from build123d import *

# Parameters (mm, degrees)
SKETCH_1_W          = 20
SKETCH_1_H          = 19.5
EXTRUDE_1_DEPTH     = 4
SKETCH_2_W          = 20
SKETCH_2_H          = 5
EXTRUDE_2_DEPTH     = 21
SKETCH_3_W          = 9.5
SKETCH_3_H          = 7
EXTRUDE_3_DEPTH     = 3
SKETCH_4_W          = 9.5
SKETCH_4_H          = 7
EXTRUDE_4_DEPTH     = 3
SKETCH_5_R          = 2.6
CUT_EXTRUDE_1_DEPTH = 36.089172119
SKETCH_6_R          = 2.6
CUT_EXTRUDE_2_DEPTH = 30.791987178


with BuildPart() as part:
    # 草图1 → 凸台-拉伸1 (new body)
    with BuildSketch(Plane.XY):
        Rectangle(SKETCH_1_W, SKETCH_1_H)
    extrude(amount=EXTRUDE_1_DEPTH)

    # 草图2 → 凸台-拉伸2 (add)
    with BuildSketch(Plane.XY.offset(4)):
        with Locations((0, 7.25)):
            Rectangle(SKETCH_2_W, SKETCH_2_H)
        with Locations((0, -7.25)):
            Rectangle(SKETCH_2_W, SKETCH_2_H)
    extrude(amount=EXTRUDE_2_DEPTH)

    # 草图3 → 凸台-拉伸3 (add)
    with BuildSketch(Plane(origin=(0, 9.75, 0), x_dir=(1, 0, 0), z_dir=(0, 1, 0))):
        with Locations((0, -8.5)):
            Rectangle(SKETCH_3_W, SKETCH_3_H)
    extrude(amount=EXTRUDE_3_DEPTH)

    # 草图4 → 凸台-拉伸4 (add)
    with BuildSketch(Plane.XZ.offset(9.75)):
        with Locations((0, 8.5)):
            Rectangle(SKETCH_4_W, SKETCH_4_H)
    extrude(amount=EXTRUDE_4_DEPTH)

    # 草图5 → 切除-拉伸1 (cut, through all)
    with BuildSketch(Plane(origin=(0, 9.75, 0), x_dir=(1, 0, 0), z_dir=(0, 1, 0))):
        with Locations(Location((0, -19, 0), (0, 0, 270))):
            Circle(SKETCH_5_R)
    extrude(amount=-CUT_EXTRUDE_1_DEPTH, mode=Mode.SUBTRACT)

    # 草图6 → 切除-拉伸2 (cut, through all)
    with BuildSketch(Plane(origin=(0, 0, 0), x_dir=(-1, 0, 0), z_dir=(0, 0, -1))):
        Circle(SKETCH_6_R)
    extrude(amount=-CUT_EXTRUDE_2_DEPTH, mode=Mode.SUBTRACT)


solid = part.part
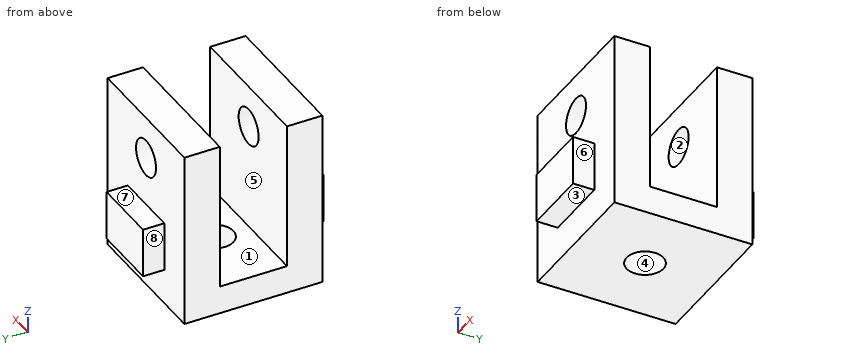
Model file for the job. Use its own axes, mm. Face numbers are marked on the shaded views. A direction names the side the tool comes from. Coordinates: 2 decimals unless noted, no trailing zeros. Loops run counter-clockwise (first coordinate to the right, second up) from the corner with the lowest first, then second, coordinate; pieces in that order, holes last. Notation, with made-up numbers: (3, 81.5) -> (12, 81.5) arc R30 ccw to (12, 110.5) -> close; hole circle Ø3 at (-7.75, 80.5). An arc over 180 degrees is marked (long way). Use one line per item in the form item = value. Start each with the question number.
(1) Flat gauge pins, fed straight in: pin 1 (6 mm diameter, centred on x = 8, z = 17.5, fed in from +Y); pin 2 (0.9 mm diameter, centred on y = 10.5, z = 7.5, fed in from +X); pin 3 (1.5 mm diameter, centred on x = 0.5, y = 11.5, fed in from +Z); pin 4 (1 mm diameter, centred on x = -0.5, z = 20, fed in from -Y). Where does each tip first touch, or does it go through?
(2) Tool access for the marked faces 4, 5, 6, 7 and 8: list every direction of +Z, -Z, +X, -X, +Y, -Y with a clear straight run to the whole face (end or side of a thin tool).
(3) Pull direction Z, two halves, no side cores. Call the marked faces 1, 2 and 3: pulls with the +Z half, pulls with the -Z half, needs draft (parallel to the pull), parting line crosses it, or undercut.
(4) Cut at D-D on z = 3. Give the cut face in (x, y), and give its area (3 significant figures).
(5) Probe probe 1 along X at (y, z) = (-6.45, 19); probe 2 along Y at (x, z) = (-4, 5.25); probe 3 along Y at (x, z) = (-8, 24.25). List the from-to ranges inside material, lowest first. Write a range as from..to.
(6) Cut at B-B on x = 0. Give the cut face in (y, z).
(7) Cut at C-C on y = 0. Give the cut face in (x, z).
(8) Cut at A-A on z = 19. Give the cut face in (x, y), and give its area (3 significant figures).
Values:
q1.pin_1 = 9.75
q1.pin_2 = 4.75
q1.pin_3 = 12
q1.pin_4 = through
q2.face_4 = +Z, -Z
q2.face_5 = +Z, +X, -X
q2.face_6 = +Z, -Z, +X, -Y
q2.face_7 = +Z, +X, -X, +Y
q2.face_8 = +Z, -Z, -X, +Y
q3.face_1 = pulls with the +Z half
q3.face_2 = undercut
q3.face_3 = pulls with the -Z half
q4.outline = (-10, -9.75) -> (10, -9.75) -> (10, 9.75) -> (-10, 9.75) -> close; hole circle Ø5.2 at (0, 0)
q4.area = 369 mm2
q5.probe_1 = -10..-2.6, 2.6..10
q5.probe_2 = -12.75..-4.75, 4.75..12.75
q5.probe_3 = -9.75..-4.75, 4.75..9.75
q6.outline = (-12.75, 5) -> (-9.75, 5) -> (-9.75, 0) -> (-2.6, 0) -> (-2.6, 4) -> (-4.75, 4) -> (-4.75, 16.4) -> (-9.75, 16.4) -> (-9.75, 12) -> (-12.75, 12) -> close; (-9.75, 21.6) -> (-4.75, 21.6) -> (-4.75, 25) -> (-9.75, 25) -> close; (2.6, 0) -> (9.75, 0) -> (9.75, 5) -> (12.75, 5) -> (12.75, 12) -> (9.75, 12) -> (9.75, 16.4) -> (4.75, 16.4) -> (4.75, 4) -> (2.6, 4) -> close; (4.75, 21.6) -> (9.75, 21.6) -> (9.75, 25) -> (4.75, 25) -> close
q7.outline = (-10, 0) -> (-2.6, 0) -> (-2.6, 4) -> (-10, 4) -> close; (2.6, 0) -> (10, 0) -> (10, 4) -> (2.6, 4) -> close
q8.outline = (-10, -9.75) -> (-2.6, -9.75) -> (-2.6, -4.75) -> (-10, -4.75) -> close; (-10, 4.75) -> (-2.6, 4.75) -> (-2.6, 9.75) -> (-10, 9.75) -> close; (2.6, -9.75) -> (10, -9.75) -> (10, -4.75) -> (2.6, -4.75) -> close; (2.6, 4.75) -> (10, 4.75) -> (10, 9.75) -> (2.6, 9.75) -> close
q8.area = 148 mm2
